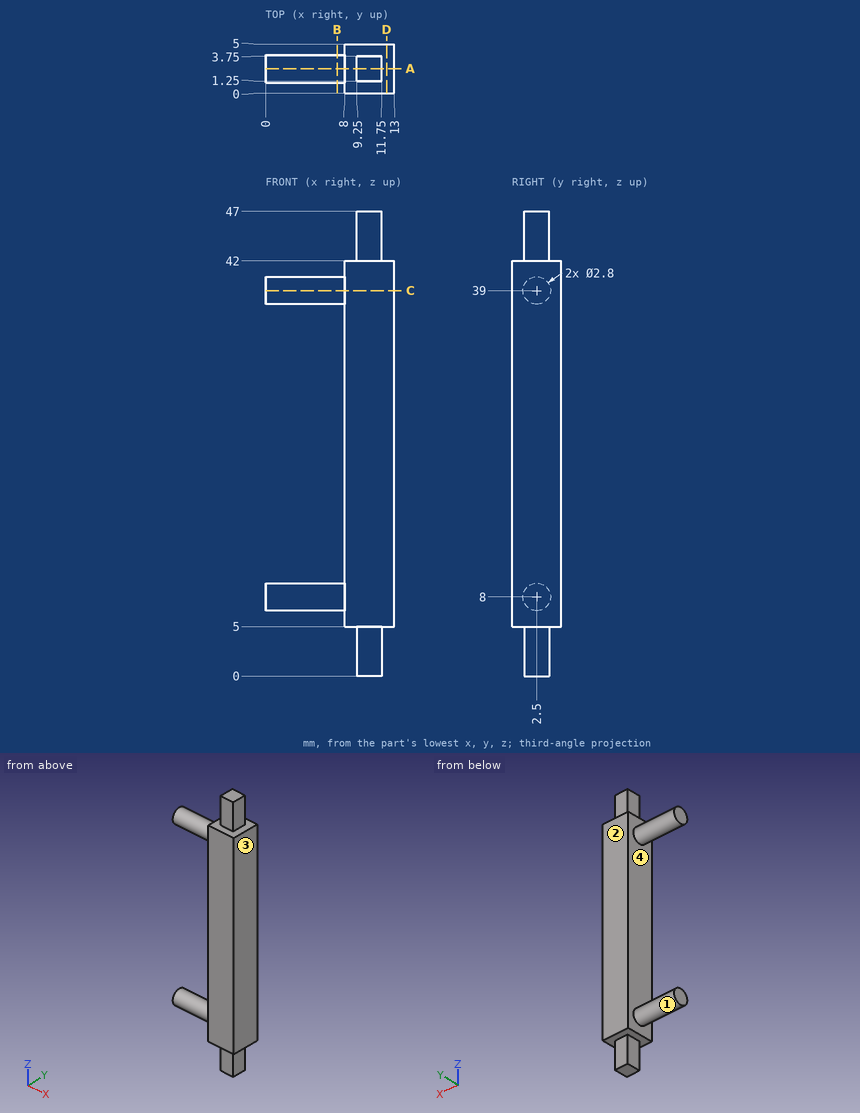
Can you work these out from the drawing? Everything is in mm from the part's minimum corner. A direction names the side the tool comes from. Give positions to 0.01 mm unless a question says otherwise; leave off trailing zeros. Loops run counter-clockwise (first coordinate to the right, second up) from the corner with the lowest first, then second, coordinate; pieces in that order, holes last. Notation, with made-up numbers: M -13.75,-6 L 3.25,-6 A23 ccw 3.25,5 Z; hole C 24.25,71.5 d7. An arc over 180 degrees is marked long. Put each result on its own line as item: value. Start each with the question number.
(1) I want a section at A-A on y = 2.5. Please give me the cut outline in (x, z).
(2) I need wall thicknesses on line 1 along Z through (x, y) = (1.5, 2.5); line 2 along Z through (x, y) = (10, 1.2); line 3 along X through (y, z) = (3.75, 23.5). Which ranges of each line are inside material? Lowest first, please. Write a range as [from, to].
(3) I want a section at B-B on x = 7.25. Please give me the cut outline in (y, z), then the cut area to 3 significant figures.
(4) Will these pins go through, and if not, where does the flat tip stop? pin 1 Ø1.2 at (y, z) = (2.5, 43.5) entering from -X; pin 2 Ø1.5 at (y, z) = (3, 27) entering from -X; pin 3 Ø2 at (x, z) = (11, 15) entering from -Y; pin 4 Ø2 at (y, z) = (3, 45) entering from +X.
(5) I want a section at C-C on z = 39. Please give me the cut outline in (x, y), then the cut area to 3 significant figures.
(6) For the marked faces 1 and 2, which set-ups out of +Z, -Z, +X, -X, +Y, -Y let a thin tool reach every point of the face, with its end or its side?
(7) If we mould it in two halves opening along Z, with no side actions, what happens to the marked faces 3 and 4? For each: +Z half, -Z half, draft (parallel to the pull), parting line (faces both ways), or undercut.
(8) I want a section at D-D on x = 12.25. Please give me the cut outline in (y, z).
Answer block:
1. outline: M 0,6.6 L 8,6.6 L 8,5 L 9.25,5 L 9.25,0 L 11.75,0 L 11.75,5 L 13,5 L 13,42 L 11.75,42 L 11.75,47 L 9.25,47 L 9.25,42 L 8,42 L 8,40.4 L 0,40.4 L 0,37.6 L 8,37.6 L 8,9.4 L 0,9.4 Z
2. line 1: [6.6, 9.4], [37.6, 40.4]
2. line 2: [5, 42]
2. line 3: [8, 13]
3. outline: C 2.5,8 d2.8; C 2.5,39 d2.8
3. area: 12.3 mm^2
4. pin 1: x = 9.25
4. pin 2: x = 8
4. pin 3: y = 0
4. pin 4: x = 11.75
5. outline: M 0,1.1 L 8,1.1 L 8,0 L 13,0 L 13,5 L 8,5 L 8,3.9 L 0,3.9 Z
5. area: 47.4 mm^2
6. face 1: -X
6. face 2: +Z, -Z, +X, -X, +Y
7. face 3: draft
7. face 4: undercut
8. outline: M 0,5 L 5,5 L 5,42 L 0,42 Z
